Check sheet for the modelled part. Datum: model origin and axes. Units: mm. Give positions to 0.01 mm unless a question says otherwise; leave off trailing zeros. Order: outer loops, then holes, each group sorted by start corner. A loop starts at its lowest first (then second) coordinate and runs counter-clockwise, first axis right, second up. Notation, with made-up numbers: (53.5, 39.25) - (102.5, 39.25) arc R14 cw to (102.5, 48.25) - close; hole circle Ø5 at (-0.5, 40.5). An arc over 180 degrees is marked (long way). Answer in a Markdown table with one row per item.
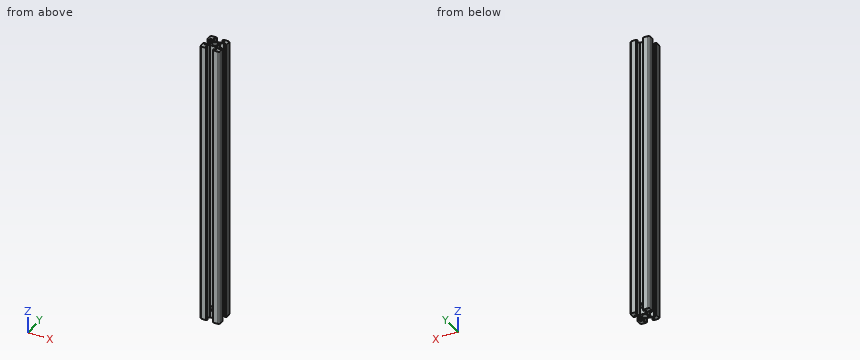
from build123d import *

# Parameters (mm, degrees)
SKETCH_1_R          = 2.55
EXTRUDE_1_DEPTH     = 300
SKETCH_2_R          = 3
CUT_EXTRUDE_1_DEPTH = 301.83217913
SKETCH_3_R          = 3
CUT_EXTRUDE_2_DEPTH = 301.83217923


with BuildPart() as part:
    # 草图1 → 凸台-拉伸1 (new body)
    with BuildSketch(Plane.XY):
        with BuildLine():
            Line((-3.9, 2.839339828), (-6.560660172, 5.5))
            Line((-6.560660172, 5.5), (-8.2, 5.5))
            Line((-8.2, 5.5), (-8.2, 3.1))
            Line((-8.2, 3.1), (-9.45, 3.1))
            Line((-9.45, 3.1), (-9.45, 3.65))
            Line((-9.45, 3.65), (-10, 3.65))
            Line((-10, 3.65), (-10, 8.5))
            ThreePointArc((-10, 8.5), (-9.560660172, 9.560660172), (-8.5, 10))
            Line((-8.5, 10), (-3.65, 10))
            Line((-3.65, 10), (-3.65, 9.45))
            Line((-3.65, 9.45), (-3.1, 9.45))
            Line((-3.1, 9.45), (-3.1, 8.2))
            Line((-3.1, 8.2), (-5.5, 8.2))
            Line((-5.5, 8.2), (-5.5, 6.560660172))
            Line((-5.5, 6.560660172), (-2.839339828, 3.9))
            Line((-2.839339828, 3.9), (2.839339828, 3.9))
            Line((2.839339828, 3.9), (5.5, 6.560660172))
            Line((5.5, 6.560660172), (5.5, 8.2))
            Line((5.5, 8.2), (3.1, 8.2))
            Line((3.1, 8.2), (3.1, 9.45))
            Line((3.1, 9.45), (3.65, 9.45))
            Line((3.65, 9.45), (3.65, 10))
            Line((3.65, 10), (8.5, 10))
            ThreePointArc((8.5, 10), (9.560660172, 9.560660172), (10, 8.5))
            Line((10, 8.5), (10, 3.65))
            Line((10, 3.65), (9.45, 3.65))
            Line((9.45, 3.65), (9.45, 3.1))
            Line((9.45, 3.1), (8.2, 3.1))
            Line((8.2, 3.1), (8.2, 5.5))
            Line((8.2, 5.5), (6.560660172, 5.5))
            Line((6.560660172, 5.5), (3.9, 2.839339828))
            Line((3.9, 2.839339828), (3.9, -2.839339828))
            Line((3.9, -2.839339828), (6.560660172, -5.5))
            Line((6.560660172, -5.5), (8.2, -5.5))
            Line((8.2, -5.5), (8.2, -3.1))
            Line((8.2, -3.1), (9.45, -3.1))
            Line((9.45, -3.1), (9.45, -3.65))
            Line((9.45, -3.65), (10, -3.65))
            Line((10, -3.65), (10, -8.5))
            ThreePointArc((10, -8.5), (9.560660172, -9.560660172), (8.5, -10))
            Line((8.5, -10), (3.65, -10))
            Line((3.65, -10), (3.65, -9.45))
            Line((3.65, -9.45), (3.1, -9.45))
            Line((3.1, -9.45), (3.1, -8.2))
            Line((3.1, -8.2), (5.5, -8.2))
            Line((5.5, -8.2), (5.5, -6.560660172))
            Line((5.5, -6.560660172), (2.839339828, -3.9))
            Line((2.839339828, -3.9), (-2.839339828, -3.9))
            Line((-2.839339828, -3.9), (-5.5, -6.560660172))
            Line((-5.5, -6.560660172), (-5.5, -8.2))
            Line((-5.5, -8.2), (-3.1, -8.2))
            Line((-3.1, -8.2), (-3.1, -9.45))
            Line((-3.1, -9.45), (-3.65, -9.45))
            Line((-3.65, -9.45), (-3.65, -10))
            Line((-3.65, -10), (-8.5, -10))
            ThreePointArc((-8.5, -10), (-9.560660172, -9.560660172), (-10, -8.5))
            Line((-10, -8.5), (-10, -3.65))
            Line((-10, -3.65), (-9.45, -3.65))
            Line((-9.45, -3.65), (-9.45, -3.1))
            Line((-9.45, -3.1), (-8.2, -3.1))
            Line((-8.2, -3.1), (-8.2, -5.5))
            Line((-8.2, -5.5), (-6.560660172, -5.5))
            Line((-6.560660172, -5.5), (-3.9, -2.839339828))
            Line((-3.9, -2.839339828), (-3.9, 2.839339828))
        make_face()
        Circle(SKETCH_1_R, mode=Mode.SUBTRACT)
    extrude(amount=EXTRUDE_1_DEPTH)

    # 草图2 → 切除-拉伸1 (cut, through all)
    with BuildSketch(Plane(origin=(0, 10, 0), x_dir=(1, 0, 0), z_dir=(0, 1, 0))):
        with Locations(Location((0, -10, 0), (0, 0, 198.835996158))):
            Circle(SKETCH_2_R)
    extrude(amount=-CUT_EXTRUDE_1_DEPTH, mode=Mode.SUBTRACT)

    # 草图3 → 切除-拉伸2 (cut, through all)
    with BuildSketch(Plane(origin=(10, 0, 0), x_dir=(0, 0, -1), z_dir=(1, 0, 0))):
        with Locations(Location((-140, 0, 0), (0, 0, 71.164003842))):
            Circle(SKETCH_3_R)
    extrude(amount=-CUT_EXTRUDE_2_DEPTH, mode=Mode.SUBTRACT)


solid = part.part
(1) Gauge pin test, flat ends, axial feed: P1, Ø0.6, axis at y = 9.5, z = 182.5, coming from the -X side; P2, Ø0.6, axis at y = -9.5, z = 148.5, coming from the +X side; P3, Ø3, axis at y = 2, z = 185, coming from the +X side. Record the tip position at first contact, or that the pin passes through.
Geometry says:
| item | result |
|---|---|
| P1 | x = -9.83 |
| P2 | x = 9.83 |
| P3 | x = 9.45 |
(2) Cross-section at A-A, the plane x = 0. Record the cut outline in (y, z).
Geometry says:
| item | result |
|---|---|
| outline | (-3.9, 0) - (-2.55, 0) - (-2.55, 7) - (-3.9, 7) - close; (-3.9, 13) - (-2.55, 13) - (-2.55, 138.42) arc R3 cw to (-2.55, 141.58) - (-2.55, 300) - (-3.9, 300) - close; (2.55, 0) - (3.9, 0) - (3.9, 7) - (2.55, 7) - close; (2.55, 13) - (3.9, 13) - (3.9, 300) - (2.55, 300) - (2.55, 141.58) arc R3 cw to (2.55, 138.42) - close |
(3) Cross-section at B-B, the plane y = 0. Record the cut outline in (x, z).
Geometry says:
| item | result |
|---|---|
| outline | (-3.9, 0) - (-2.55, 0) - (-2.55, 8.42) arc R3 cw to (-2.55, 11.58) - (-2.55, 137) - (-3.9, 137) - close; (-3.9, 143) - (-2.55, 143) - (-2.55, 300) - (-3.9, 300) - close; (2.55, 0) - (3.9, 0) - (3.9, 137) - (2.55, 137) - (2.55, 11.58) arc R3 cw to (2.55, 8.42) - close; (2.55, 143) - (3.9, 143) - (3.9, 300) - (2.55, 300) - close |
(4) Thickness scan on L1, parallel to Y at x = 0, z = 5.5; L2, parallel to Y at x = 1.75, z = 140. Record the ranges inside material, lowest first.
Geometry says:
| item | result |
|---|---|
| L1 | -3.9 to -2.55, 2.55 to 3.9 |
| L2 | -3.9 to -3, 3 to 3.9 |
